Input: dimensioned drawing with shaded views. Units: mm. Origin: part minimum x, y, z. A direction names the side the tool comes from. Give positions to 0.01 mm unless a question says otherwise; leave off trailing zeros. Order: outer loops, then holes, each group sorted by start corner. A loop starts at its lowest first (then second) coordinate and runs counter-clockwise, first axis right, second up. Notation, with made-up numbers: (-30, 58.5) -> (18, 58.5) arc R18 ccw to (18, 82.5) -> close; hole circle Ø3 at (-8, 52). An arc over 180 degrees is marked (long way). One line per question, with ' | ' between items. Start each with the question number.
(1) Mould query, pull axis X, two halves, no side actions, for the marked faces 1, 2 and 3. Classes: +X half, -X half, draft (parallel to the pull), parting line (faces both ways), or undercut.
(2) Section D-D (z = 1.5). Return loops of the section in (x, y) (1 decimal).
(3) First-contact query: pin 1 Ø2 at (y, z) = (2.5, 3.5) entering from +X; pin 2 Ø1 at (x, y) = (4, 1.5) entering from -Z; pin 3 Ø1.5 at (x, y) = (5, 3) entering from -Z. Flat tips, straight axial feed; report the tip coordinate or a pass-through.
(4) Section C-C (y = 6.75). Return loops of the section in (x, z).
(5) Set-up query: the marked faces 4 and 5. Return all of +Z, -Z, +X, -X, +Y, -Y with unobstructed straight access to the full face (end or side cutting, diameter ignored); none if empty.
(6) Ray query, L1, parallel to Z at x = 3, y = 6; L2, parallel to Z at x = 1.25, y = 2.5; L3, parallel to X at y = 1.25, z = 3. Return the intervals inside material, ascending.
(7) Section B-B (z = 3.1). Return loops of the section in (x, y).
(8) Section A-A (x = 3.1). Return loops of the section in (y, z).
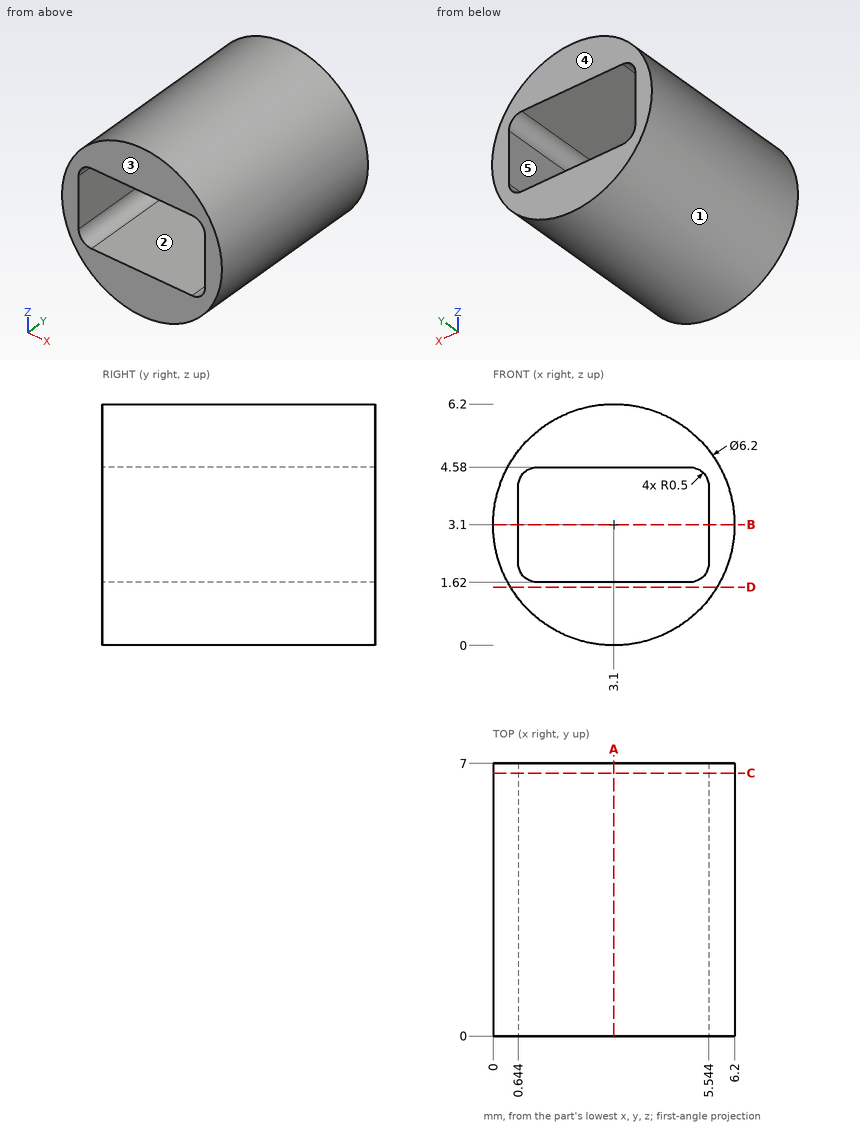
Response:
1) face 1: parting line | face 2: undercut | face 3: draft
2) outline: (0.4, 0) -> (5.8, 0) -> (5.8, 7) -> (0.4, 7) -> close
3) pin 1: stops at x = 6.2 | pin 2: stops at z = 0.03 | pin 3: stops at z = 0.22
4) outline: circle Ø6.2 at (3.1, 3.1); hole (0.64, 2.12) arc R0.5 ccw to (1.14, 1.62) -> (5.04, 1.62) arc R0.5 ccw to (5.54, 2.12) -> (5.54, 4.08) arc R0.5 ccw to (5.04, 4.58) -> (1.14, 4.58) arc R0.5 ccw to (0.64, 4.08) -> close
5) face 4: +Z, -Z, +X, -X, +Y | face 5: +Y, -Y
6) L1: z = 0 to 1.62, 4.58 to 6.2 | L2: z = 0.61 to 1.62, 4.58 to 5.59 | L3: x = 0 to 0.64, 5.54 to 6.2
7) outline: (0, 0) -> (0.64, 0) -> (0.64, 7) -> (0, 7) -> close; (5.54, 0) -> (6.2, 0) -> (6.2, 7) -> (5.54, 7) -> close
8) outline: (0, 0) -> (7, 0) -> (7, 1.62) -> (0, 1.62) -> close; (0, 4.58) -> (7, 4.58) -> (7, 6.2) -> (0, 6.2) -> close
